```python
from build123d import *

# Parameters (mm, degrees)
SKETCH031_W   = 90
SKETCH031_H   = 140
SKETCH031_R   = 11.05
SKETCH031_R_2 = 2.75
SKETCH031_R_3 = 6.1
SKETCH031_R_4 = 6.05
SKETCH031_R_5 = 3.55
PAD014_DEPTH  = 3
SKETCH032_W   = 85
SKETCH032_H   = 120
SKETCH032_W_2 = 82
SKETCH032_H_2 = 117
PAD015_DEPTH  = 30
FILLET014_R   = 5


with BuildPart() as part:
    # Sketch031 → Pad014 (new body)
    with BuildSketch(Plane.XY):
        Rectangle(SKETCH031_W, SKETCH031_H)
        with Locations((-22.5, -40)):
            Circle(SKETCH031_R, mode=Mode.SUBTRACT)
        with Locations((-39, 65)):
            Circle(SKETCH031_R_2, mode=Mode.SUBTRACT)
        with Locations((39, 65)):
            Circle(SKETCH031_R_2, mode=Mode.SUBTRACT)
        with Locations((39, -65)):
            Circle(SKETCH031_R_2, mode=Mode.SUBTRACT)
        with Locations((-39, -65)):
            Circle(SKETCH031_R_2, mode=Mode.SUBTRACT)
        with Locations((-22.5, -5)):
            Circle(SKETCH031_R_3, mode=Mode.SUBTRACT)
        with Locations((-27.5, 48)):
            Circle(SKETCH031_R_4, mode=Mode.SUBTRACT)
        with Locations((0, 48)):
            Circle(SKETCH031_R_4, mode=Mode.SUBTRACT)
        with Locations((27.5, 48)):
            Circle(SKETCH031_R_4, mode=Mode.SUBTRACT)
        with Locations((27.5, -48)):
            Circle(SKETCH031_R_5, mode=Mode.SUBTRACT)
        with Locations((27.5, -23)):
            Circle(SKETCH031_R_5, mode=Mode.SUBTRACT)
        with Locations((27.5, 2)):
            Circle(SKETCH031_R_5, mode=Mode.SUBTRACT)
        with Locations((27.5, 27)):
            Circle(SKETCH031_R_5, mode=Mode.SUBTRACT)
        with Locations((-22.5, 25)):
            Circle(SKETCH031_R_4, mode=Mode.SUBTRACT)
    extrude(amount=PAD014_DEPTH)

    # Sketch032 (on Face19 of Pad014) → Pad015 (join)
    with BuildSketch(Plane(origin=(0, 0, 0), x_dir=(1, 0, 0), z_dir=(0, 0, -1))):
        Rectangle(SKETCH032_W, SKETCH032_H)
        Rectangle(SKETCH032_W_2, SKETCH032_H_2, mode=Mode.SUBTRACT)
    extrude(amount=PAD015_DEPTH)

    # Fillet014
    fillet014_edges = [part.edges().sort_by_distance(p)[0] for p in [
        (45, 70, 1.5),
        (-45, 70, 1.5),
        (45, -70, 1.5),
        (-45, -70, 1.5),
    ]]
    fillet(fillet014_edges, radius=FILLET014_R)


solid = part.part
```
CAD build for the part. Positions are in the model's coordinates, mm. A direction names the side the tool comes from. Coordinates: 2 decimals unless noted, no trailing zeros. Write each loop counter-clockwise with the first axis right and the second up, starting at its lowest first coordinate (ties: lowest second). Pieces come first, ordered by that corner, then holes.
(1) Cut at D-D, the plane y = 16. List the corners of the cut face in (x, z).
(2) Flat gauge pins, fed straight in: pin 1 (10 mm diameter, centred on x = -3.5, z = -15, fed in from +Y); pin 2 (9 mm diameter, centred on x = -39, y = -65, fed in from +Z); pin 3 (10 mm diameter, centred on x = -25, z = -14.5, fed in from -Y); pin 4 (3 mm diameter, centred on y = -35, z = -13.5, fed in from -X). Where does each tip first touch, or does it go through?
(3) Cut at B-B, the plane y = 48. List the corners of the cut face in (x, z).
(4) Drill centre lines: probe 1 along X at (y, z) = (-13, -6); probe 2 along Y at (x, z) = (22, -4.5); probe 3 along Z at (x, y) = (33, 4). Where is each one in solid material? Low to high.
(5) Two-plate mould, pull along X, no slides. Class faces 1 (the face through (-1, -58.5, -15)), 2 (the face through (-31.96, 52.09, 1.48)), 3 (the face through (42.5, 1, -15)), 4 (the face through (-1, 70, 1)): +X half, -X half, draft (parallel to the pull), parting line (faces both ways), or undercut.
(6) 3-axis set-ups, long thin cutter, end or side, ignore diameter. For faces 5 (the face through (23.953, 27.156, 1.479)), 6 (the face through (-1, 60, -15)), 7 (the face through (-1, -60, -15)), 8 (the face through (-42.5, 1, -15)), 9 (the face through (-41, 1, -15)): which of +Z, -Z, +X, -X, +Y, -Y reach the whole face in a straight line?
(7) Cut at C-C, the plane z = -2.5. List the corners of the cut face in (x, y).
(8) Cut at A-A, the plane x = 27.5. Count the separate pieces of the cut face and the enclosed holes in it, and give its area (4 significant figures).
Geometry says:
1. outline: (-45, 0) - (-42.5, 0) - (-42.5, -30) - (-41, -30) - (-41, 0) - (41, 0) - (41, -30) - (42.5, -30) - (42.5, 0) - (45, 0) - (45, 3) - (-45, 3) - close
2. pin 1: stops at y = 60
2. pin 2: stops at z = 3
2. pin 3: stops at y = -60
2. pin 4: stops at x = -42.5
3. outline: (-45, 0) - (-42.5, 0) - (-42.5, -30) - (-41, -30) - (-41, 0) - (-33.55, 0) - (-33.55, 3) - (-45, 3) - close; (-21.45, 0) - (-6.05, 0) - (-6.05, 3) - (-21.45, 3) - close; (6.05, 0) - (21.45, 0) - (21.45, 3) - (6.05, 3) - close; (33.55, 0) - (41, 0) - (41, -30) - (42.5, -30) - (42.5, 0) - (45, 0) - (45, 3) - (33.55, 3) - close
4. probe 1: x = -42.5 to -41, 41 to 42.5
4. probe 2: y = -60 to -58.5, 58.5 to 60
4. probe 3: z = 0 to 3
5. face 1: undercut
5. face 2: undercut
5. face 3: +X half
5. face 4: draft
6. face 5: +Z, -Z
6. face 6: -Z, +X, -X, +Y
6. face 7: -Z, +X, -X, -Y
6. face 8: -Z, -X, +Y, -Y
6. face 9: -Z
7. outline: (-42.5, -60) - (42.5, -60) - (42.5, 60) - (-42.5, 60) - close; hole (-41, -58.5) - (41, -58.5) - (41, 58.5) - (-41, 58.5) - close
8. separate pieces: 6
8. enclosed holes: 0
8. area: 388.5 mm2
